from build123d import *

# Parameters (mm, degrees)
EXTRUDE_1_DEPTH = 10
FILLET_1_R      = 0.2


with BuildPart() as part:
    # Эскиз1 → Бобышка-Вытянуть1 (new body, symmetric)
    with BuildSketch(Plane.XY):
        Polygon((5, 0), (-5, 0), (-5, -4.3), (-9.75, -4.3), (-9.75, -6.8), (-5, -10.5), (5, -10.5), (9.75, -6.8), (9.75, -4.3), (5, -4.3), align=None)
    extrude(amount=EXTRUDE_1_DEPTH, both=True)

    # Эскиз4 → Отверстие обработанное метчиком M44 (revolve, cut)
    with BuildSketch(Plane(origin=(0, 0, 0), x_dir=(0, 0, 1), z_dir=(1, 0, 0))):
        Polygon((0, 0), (0, 10.5), (2.15, 10.5), (1.65, 10), (1.65, 0.5), (2.15, 0), align=None)
    revolve(axis=Axis((0, 6.35, 0), (0, -1, 0)), mode=Mode.SUBTRACT)

    # Скругление1
    fillet_1_edges = [part.edges().sort_by_distance(p)[0] for p in [
        (-5, 0, 0),
        (5, 0, 0),
        (5, -4.3, 0),
        (9.75, -4.3, 0),
        (5, -10.5, 0),
        (-5, -10.5, 0),
        (-9.75, -4.3, 0),
        (-5, -4.3, 0),
    ]]
    fillet(fillet_1_edges, radius=FILLET_1_R)


solid = part.part
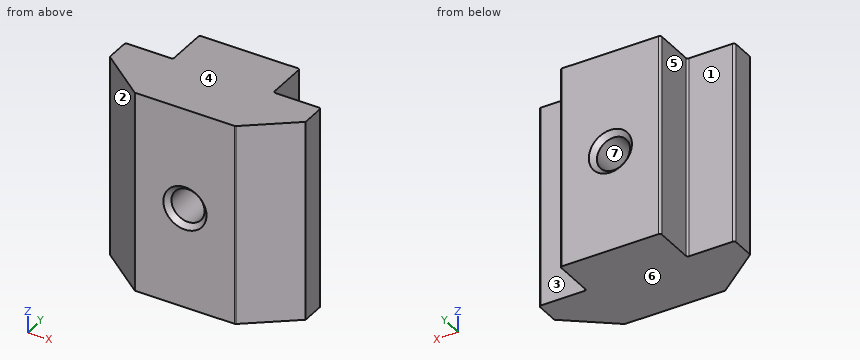
The model under review builds one solid part; all positions refer to its coordinate system, in mm. Face numbers are marked on the shaded views. A direction names the side the tool comes from. Round coordinates to 2 decimals unless told otherwise and drop trailing zeros. Write each loop counter-clockwise with the first axis right and the second up, starting at its lowest first coordinate (ties: lowest second). Pieces come first, ordered by that corner, then holes. Notation, with made-up numbers: M 41,68 L 69,68 A6 cw 69,76 Z; hole C 6,-30 d6. An arc over 180 degrees is marked long. Use a Markdown table: item, result. Add a question column.
Q1. Machinability: for the marked faces 1, 2 and 3, which of the approach directions +Z, -Z, +X, -X, +Y, -Y give a long, thin tool a straight path to every point of the face, cutting with its end or side? Answer none if there is none.
Q2. We need section D-D, the plane z = -4.75. State the section outline as (x, y) points.
Q3. We need section B-B, the plane y = -6. State the section outline as (x, z) points, plus the area to 3 significant figures.
Q4. We need section C-C, the plane z = 0. State the section outline as (x, y) points.
Q5. We need section A-A, the plane x = 0. State the section outline as (y, z) points.
Q6. Insertion check: pin 1 (3 mm diameter, centred on y = -1, z = -1, fed in from +X); pin 2 (2 mm diameter, centred on x = -7.5, z = 0, fed in from +Y); pin 3 (1.2 mm diameter, centred on y = -2, z = 1.5, fed in from -X). Each pin has a flat end and moves straight along its axis. Give the tip position at first contact, or say it passes through.
Q7. The part is to be moulded in two halves that separate along Z. For the marked faces 4, 5, 6 and 7, say which applies: pulls with the +Z half, pulls with the -Z half, needs draft (parallel to the pull), parting line crosses it, or undercut.
Q8. To check wall thickness, follow line 1 (Z direction, x = 0, y = -3.5); line 2 (X direction, y = -4.5, z = 0); line 3 (X direction, y = -2, z = -3.25). State the ranges of each line that lie inside material, in increasing order.
Findings below:
| question | item | result |
|---|---|---|
| 1 | face 1 | +Z, -Z, -X, +Y |
| 1 | face 2 | +Z, -Z, -X, -Y |
| 1 | face 3 | +Z, -Z, +X, +Y |
| 2 | outline | M -9.75,-6.8 L -5.05,-10.46 A0.2 ccw -4.93,-10.5 L 4.93,-10.5 A0.2 ccw 5.05,-10.46 L 9.75,-6.8 L 9.75,-4.5 A0.2 ccw 9.55,-4.3 L 5.2,-4.3 A0.2 cw 5,-4.1 L 5,-0.2 A0.2 ccw 4.8,0 L -4.8,0 A0.2 ccw -5,-0.2 L -5,-4.1 A0.2 cw -5.2,-4.3 L -9.55,-4.3 A0.2 ccw -9.75,-4.5 Z |
| 3 | outline | M -9.75,-10 L 9.75,-10 L 9.75,10 L -9.75,10 Z; hole C 0,0 d3.3 |
| 3 | area | 381 mm² |
| 4 | outline | M -9.75,-6.8 L -5.05,-10.46 A0.2 ccw -4.93,-10.5 L -2.15,-10.5 L -1.65,-10 L -1.65,-0.5 L -2.15,0 L -4.8,0 A0.2 ccw -5,-0.2 L -5,-4.1 A0.2 cw -5.2,-4.3 L -9.55,-4.3 A0.2 ccw -9.75,-4.5 Z; M 1.65,-10 L 2.15,-10.5 L 4.93,-10.5 A0.2 ccw 5.05,-10.46 L 9.75,-6.8 L 9.75,-4.5 A0.2 ccw 9.55,-4.3 L 5.2,-4.3 A0.2 cw 5,-4.1 L 5,-0.2 A0.2 ccw 4.8,0 L 2.15,0 L 1.65,-0.5 Z |
| 5 | outline | M -10.5,-10 L 0,-10 L 0,-2.15 L -0.5,-1.65 L -10,-1.65 L -10.5,-2.15 Z; M -10.5,2.15 L -10,1.65 L -0.5,1.65 L 0,2.15 L 0,10 L -10.5,10 Z |
| 6 | pin 1 | stops at x = 5 |
| 6 | pin 2 | stops at y = -4.3 |
| 6 | pin 3 | stops at x = -5 |
| 7 | face 4 | pulls with the +Z half |
| 7 | face 5 | needs draft |
| 7 | face 6 | pulls with the -Z half |
| 7 | face 7 | undercut |
| 8 | line 1 | z = -10 to -1.65, 1.65 to 10 |
| 8 | line 2 | x = -9.75 to -1.65, 1.65 to 9.75 |
| 8 | line 3 | x = -5 to 5 |
